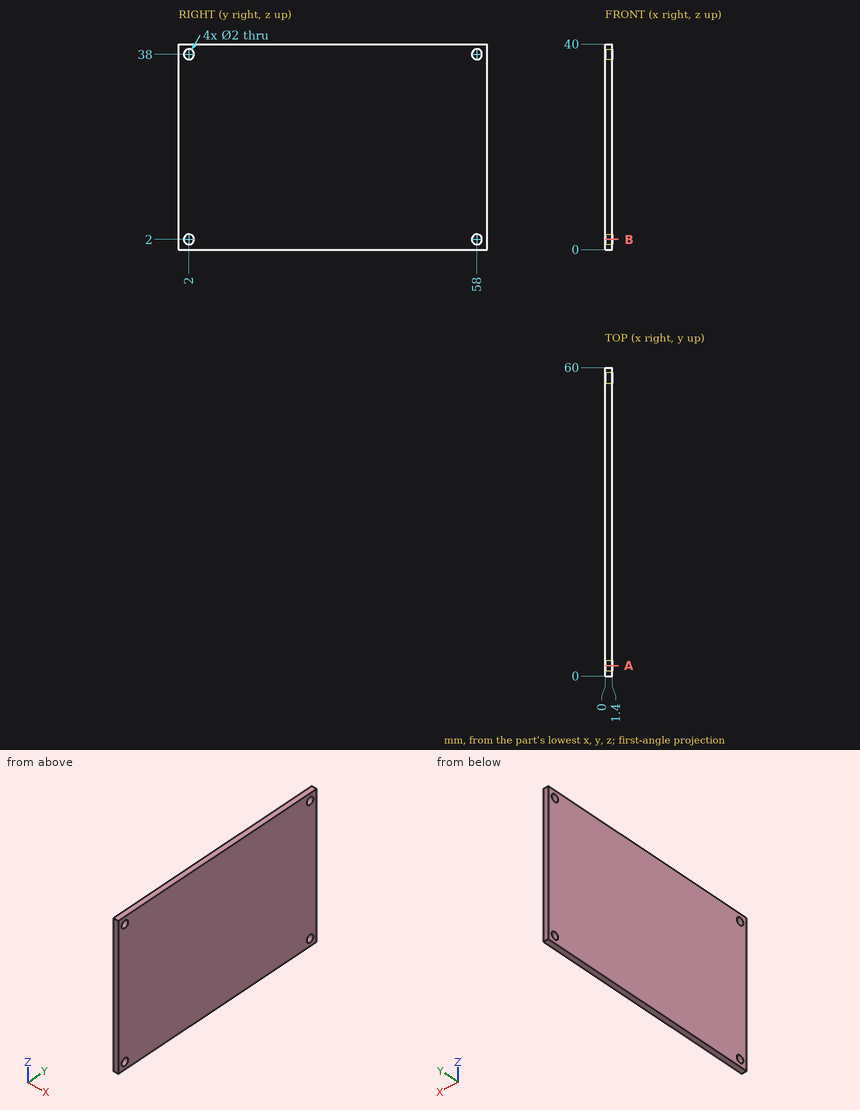
Answer from the drawing. Dimensions are ordinates in mm from the lowest x, y and z of the part. Coordinates: 2 decimals unless noted, no trailing zeros. Order: outer loops, then holes, each group sorted by start corner. A loop starts at its lowest first (then second) coordinate and runs counter-clockwise, first axis right, second up. Notation, with made-up numbers: (83, -10.5) - (91, -10.5) arc R23 ccw to (91, 2.5) - close; hole circle Ø3 at (-35, 28.5). An arc over 180 degrees is marked (long way). Use one line per item in the form item = value.
(1) Section B-B, the plane z = 2 is taken. Give the vertices of the cut face in (x, y).
Computed values:
outline = (0, 0) - (1.4, 0) - (1.4, 1) - (0, 1) - close; (0, 3) - (1.4, 3) - (1.4, 57) - (0, 57) - close; (0, 59) - (1.4, 59) - (1.4, 60) - (0, 60) - close
(2) Given pin 1 Ø1.8 at (y, z) = (2, 38) entering from -X (1 decimal); pin 2 Ø3 at (y, z) = (58, 38) entering from -X, each flat-ended and moving along its own axis, determine where each tip first touches the part or whether it passes through.
Computed values:
pin_1 = through
pin_2 = 0
(3) Section A-A, the plane y = 2 is taken. Give the vertices of the cut face in (x, z).
Computed values:
outline = (0, 0) - (1.4, 0) - (1.4, 1) - (0, 1) - close; (0, 3) - (1.4, 3) - (1.4, 37) - (0, 37) - close; (0, 39) - (1.4, 39) - (1.4, 40) - (0, 40) - close
(4) Straight lines are drawn through the part: L1, parallel to Z at x = 0.9, y = 2; L2, parallel to Y at x = 0.6, z = 38. For each, find the intervals that lie inside material, in ascending order.
Computed values:
L1 = 0 to 1, 3 to 37, 39 to 40
L2 = 0 to 1, 3 to 57, 59 to 60
